Can you work these out from the model? Positions are in its coordinate system, mm. A direction names the side the tool comes from. Give positions to 0.01 mm unless a question says otherwise; leave off trailing zeros. Write each loop counter-clockwise with the first axis right and the second up, starting at its lowest first coordinate (ties: lowest second). Pieces come first, ordered by that corner, then holes. Notation, with made-up numbers: (61, 53.5) - (107, 53.5) arc R33 ccw to (107, 82.5) - close; hole circle Ø2 at (71, 34). An arc over 180 degrees is marked (long way). Use a Markdown table: item, result. Add a question column.
```python
from build123d import *

# Parameters (mm, degrees)
STACK_CONNECTION_DEPTH       = 1.5875
EDGE_FLANGE1_DEPTH           = 30
EDGE_FLANGE2_STRIP_W         = 7.8232
EDGE_FLANGE2_STRIP_H         = 1.5875
EDGE_FLANGE2_STRIP_CUT_DEPTH = 30
EDGE_FLANGE2_DEPTH           = 30
SKETCH13_R                   = 4.7625
CUT_EXTRUDE1_DEPTH           = 57.330329085


# Sheet-metal steps are written as plain solids
with BuildPart() as part:
    # Sketch2 → Stack Connection (new body)
    with BuildSketch(Plane(origin=(0, 0, 0), x_dir=(1, 0, 0), z_dir=(0, 1, 0))):
        Polygon((-22.5, 0), (22.5, 0), (22.5, -9), (7.5, -17.6), (-22.5, -17.6), (-22.5, -9), align=None)
    extrude(amount=-STACK_CONNECTION_DEPTH)

    # Edge-Flange1 section (across the edge) → Edge-Flange1 (add)
    with BuildSketch(Plane(origin=(7.5, -1.5875, 18.3366), x_dir=(0, 0, -1), z_dir=(-1, 0, 0))):
        with BuildLine():
            Line((-1.5875, 0.7366), (-1.5875, 31.5259))
            Line((-1.5875, 31.5259), (0, 31.5259))
            Line((0, 31.5259), (0, 0.7366))
            ThreePointArc((0, 0.7366), (0.215745145, 0.215745145), (0.7366, 0))
            Line((0.7366, 0), (0.7366, -1.5875))
            ThreePointArc((0.7366, -1.5875), (-0.90678687, -0.90678687), (-1.5875, 0.7366))
        make_face()
    extrude(amount=EDGE_FLANGE1_DEPTH)

    # Edge-Flange2 strip (across the edge) → Edge-Flange2 strip cut (cut)
    with BuildSketch(Plane(origin=(-22.5, -33.1134, 19.9241), x_dir=(0, 1, 0), z_dir=(1, 0, 0))):
        with Locations((-1.5875, -0.79375)):
            Rectangle(EDGE_FLANGE2_STRIP_W, EDGE_FLANGE2_STRIP_H)
    extrude(amount=EDGE_FLANGE2_STRIP_CUT_DEPTH, mode=Mode.SUBTRACT)

    # Edge-Flange2 section (across the edge) → Edge-Flange2 (add)
    with BuildSketch(Plane(origin=(-22.5, -33.1134, 19.9241), x_dir=(0, 1, 0), z_dir=(1, 0, 0))):
        with BuildLine():
            Line((0, 0.7366), (0, 20.9779))
            Line((0, 20.9779), (1.5875, 20.9779))
            Line((1.5875, 20.9779), (1.5875, 0.7366))
            ThreePointArc((1.5875, 0.7366), (1.803245145, 0.215745145), (2.3241, 0))
            Line((2.3241, 0), (2.3241, -1.5875))
            ThreePointArc((2.3241, -1.5875), (0.68071313, -0.90678687), (0, 0.7366))
        make_face()
    extrude(amount=EDGE_FLANGE2_DEPTH)

    # Sketch13 → Cut-Extrude1 (cut, through all)
    with BuildSketch(Plane(origin=(0, -31.5259, 0), x_dir=(1, 0, 0), z_dir=(0, 1, 0))):
        with Locations(Location((-12.25, -31.3693, 0), (0, 0, 270))):
            Circle(SKETCH13_R)
    extrude(amount=-CUT_EXTRUDE1_DEPTH, mode=Mode.SUBTRACT)


solid = part.part
```
Q1. Suppose I cut it at A-A (x = -12.25). Please give me the cut outline in (y, z), and give its area (3 significant figures).
Q2. Suppose I cut it at C-C (z = 24.5). Please give me the cut outline in (x, y).
Q3. If we mould it in two halves opening along Z, with no side actions, what happens to faces 1 (the cylindrical face through (-7.29, -0.663, 19.225)), 2 (the flat face through (-8, -33.113, 28)), 3 (the cylindrical face through (-12.04, -32.31, 26.61))? For each: released by +Z, released by -Z, zero draft, split by the parting line, or undercut.
Q4. Suppose I cut it at D-D (y = -6.5). Please give me the cut outline in (x, z), and give its area (3 significant figures).
Q5. On a 3-axis mill with a long thin cutter (end or side, diameter ignored), from which of +Z, -Z, +X, -X, +Y, -Y can I reach the whole of each face in a straight line? I mean faces 4 (the flat face through (0, -1.588, 9)), 5 (the flat face through (-8, -32, 40.902)), 6 (the flat face through (-7.7, -31.526, 28.7)). Say none if no direction works.
Q6. If I drill on probe 1 along Y at (x, z) = (17, 2); probe 2 along Y at (x, z) = (-6.5, 36); probe 3 along Z at (x, y) = (-8, -19.5), over which ranges is the centre line in solid material (lowest first)? Write a range as [from, to].
Q7. Suppose I cut it at B-B (x = -0.5). Please give me the cut outline in (y, z).
Q8. I'm going to push flat-ended pins straight in: P1, Ø6, axis at x = -11.5, y = -12, coming from the +Z side; P2, Ø22.5, axis at x = -0.5, z = 32.5, coming from the +Y side; P3, Ø8.5, axis at x = -2, y = -10, coming from the -Z side. Where does each tip first touch, or does it pass through?
Derived:
| question | item | result |
|---|---|---|
| 1 | outline | (-33.11, 20.66) arc R2.32 ccw to (-30.79, 18.34) - (-2.32, 18.34) arc R0.74 cw to (-1.59, 17.6) - (-1.59, 0) - (0, 0) - (0, 17.6) arc R2.32 ccw to (-2.32, 19.92) - (-30.79, 19.92) arc R0.74 cw to (-31.53, 20.66) - (-31.53, 26.61) - (-33.11, 26.61) - close; (-33.11, 36.13) - (-31.53, 36.13) - (-31.53, 40.9) - (-33.11, 40.9) - close |
| 1 | area | 97.8 mm² |
| 2 | outline | (-22.5, -33.11) - (7.5, -33.11) - (7.5, -31.53) - (-22.5, -31.53) - close |
| 3 | face 1 | released by +Z |
| 3 | face 2 | zero draft |
| 3 | face 3 | undercut |
| 4 | outline | (-22.5, 18.34) - (7.5, 18.34) - (7.5, 19.92) - (-22.5, 19.92) - close |
| 4 | area | 47.6 mm² |
| 5 | face 4 | -Z, +X, -X, -Y |
| 5 | face 5 | +Z, +X, -X, +Y, -Y |
| 5 | face 6 | +Z, +X, -X, +Y |
| 6 | probe 1 | [-1.59, 0] |
| 6 | probe 2 | [-33.11, -31.53] |
| 6 | probe 3 | [18.34, 19.92] |
| 7 | outline | (-33.11, 20.66) arc R2.32 ccw to (-30.79, 18.34) - (-2.32, 18.34) arc R0.74 cw to (-1.59, 17.6) - (-1.59, 0) - (0, 0) - (0, 17.6) arc R2.32 ccw to (-2.32, 19.92) - (-30.79, 19.92) arc R0.74 cw to (-31.53, 20.66) - (-31.53, 40.9) - (-33.11, 40.9) - close |
| 8 | P1 | z = 19.92 |
| 8 | P2 | y = -31.53 |
| 8 | P3 | z = 18.34 |
